Could you check a few things on this model? Use its own coordinates, in mm. A direction names the side the tool comes from. Give positions to 0.01 mm unless a question says otherwise; leave off trailing zeros. Write each loop counter-clockwise with the first axis right and the second up, starting at its lowest first coordinate (ties: lowest second). Pieces come first, ordered by that corner, then holes. Notation, with made-up numbers: (-16, -18) -> (38, -18) arc R18 ccw to (38, -4) -> close; hole circle Ø8 at (31, 80.25). An arc over 180 degrees is marked (long way). Write item = value, one per line. Start each with the question number.
```python
from build123d import *

# Parameters (mm, degrees)
F1_DEPTH = 19.05
F3_DEPTH = 4
F4_R     = 1.55
F5_DEPTH = 2.5


with BuildPart() as f1:
    # F0 (on Top) → F1 (new body)
    with BuildSketch(Plane.XY):
        with BuildLine():
            Line((12.7, 0), (11.7422761358, 0))
            ThreePointArc((11.7422761358, 0), (14.5035288799, 0.4316708576), (15.774, 2.921))
            ThreePointArc((15.774, 2.921), (14.5035288799, 5.4103291424), (11.7422761358, 5.842))
            Line((11.7422761358, 5.842), (12.7, 5.842))
            Line((12.7, 5.842), (12.7, 4.471))
            ThreePointArc((12.7, 4.471), (13.7960155108, 4.0170155108), (14.25, 2.921))
            ThreePointArc((14.25, 2.921), (13.7960155108, 1.8249844892), (12.7, 1.371))
            Line((12.7, 1.371), (12.7, 0))
        make_face()
        with BuildLine():
            Line((0, 1.524), (0, 0))
            Line((0, 0), (11.7422761358, 0))
            ThreePointArc((11.7422761358, 0), (9.626, 2.921), (11.7422761358, 5.842))
            Line((11.7422761358, 5.842), (0, 5.842))
            Line((0, 5.842), (0, 4.318))
            Line((0, 4.318), (8.89, 4.318))
            Line((8.89, 4.318), (8.89, 1.524))
            Line((8.89, 1.524), (0, 1.524))
        make_face()
        with BuildLine():
            ThreePointArc((11.7422761358, 5.842), (9.626, 2.921), (11.7422761358, 0))
            Line((11.7422761358, 0), (12.7, 0))
            Line((12.7, 0), (12.7, 1.371))
            ThreePointArc((12.7, 1.371), (11.15, 2.921), (12.7, 4.471))
            Line((12.7, 4.471), (12.7, 5.842))
            Line((12.7, 5.842), (11.7422761358, 5.842))
        make_face()
    extrude(amount=F1_DEPTH)

    # F2 (on face) → F3 (join)
    with BuildSketch(Plane.XY.offset(19.05)):
        with BuildLine():
            ThreePointArc((10.2538072439, 0), (14.3118476354, -0.5312524821), (16.51, 2.921))
            ThreePointArc((16.51, 2.921), (14.3118476354, 6.3732524821), (10.2538072439, 5.842))
            Line((10.2538072439, 5.842), (11.7422761358, 5.842))
            ThreePointArc((11.7422761358, 5.842), (15.774, 2.921), (11.7422761358, 0))
            Line((11.7422761358, 0), (10.2538072439, 0))
        make_face()
    extrude(amount=-F3_DEPTH)

    # F4 (on face) → F5 (cut)
    with BuildSketch(Plane.XY.offset(19.05)):
        Polygon((15.45, 4.5087132403), (12.7, 6.0964264805), (9.95, 4.5087132403), (9.95, 1.3332867597), (12.7, -0.2544264805), (15.45, 1.3332867597), align=None)
        with Locations((12.7, 2.921)):
            Circle(F4_R, mode=Mode.SUBTRACT)
    extrude(amount=-F5_DEPTH, mode=Mode.SUBTRACT)


solid = f1.part
```
(1) Imagine slicing it at D-D (y = 5). Please give me the cut outline in (x, z).
(2) Imagine slicing it at A-A (z = 13.25). Please give me the cut outline in (x, y).
(3) We'd pull the mould along Y, two halves only. Please class faces 4 (the flat face through (0, 1, 9)), 5 (the flat face through (4, 4.318, 9)), 6 (the flat face through (6, 5.842, 9)): released by +Y, released by -Y, zero draft, split by the parting line, or undercut.
(4) On a 3-axis mill with a long thin cutter (end or side, diameter ignored), from which of +Z, -Z, +X, -X, +Y, -Y can I reach the whole of each face in a straight line? I mean faces 1 (the flat face through (8.89, 3, 9)), 2 (the flat face through (10, 3, 0)), 3 (the flat face through (15.45, 3, 18)). Say none if no direction works.
(5) If I drill on line 1 along Y through (x, z) = (3.5, 6.75); line 2 along Y through (x, z) = (12.75, 3.5); line 3 along Z through (x, y) = (15.25, 4.25), over which ranges is the centre line in solid material (lowest first)? Write a range as from..to.
(6) Imagine slicing it at B-B (x = 3.25). Please give me the cut outline in (y, z).
(7) I'm going to push flat-ended pins straight in: pin 1 (4.5 mm diameter, centred on x = 5, z = 9.5, fed in from -Y); pin 2 (1 mm diameter, centred on x = 12, y = 1, fed in from +Z); pin 3 (8 mm diameter, centred on x = 8, z = 7, fed in from +Y). Where does each tip first touch, or does it pass through?
(8) Imagine slicing it at C-C (z = 17.75). Please give me the cut outline in (x, y), then the cut area to 3 significant figures.
Answers below:
q1.outline = (0, 0) -> (14.96, 0) -> (14.96, 15.05) -> (15.89, 15.05) -> (15.89, 19.05) -> (14.6, 19.05) -> (14.6, 16.55) -> (10.8, 16.55) -> (10.8, 19.05) -> (0, 19.05) -> close
q2.outline = (0, 0) -> (11.74, 0) arc R3.07 ccw (long way) to (11.74, 5.84) -> (0, 5.84) -> (0, 4.32) -> (8.89, 4.32) -> (8.89, 1.52) -> (0, 1.52) -> close; hole circle Ø3.1 at (12.7, 2.92)
q3.face_4 = zero draft
q3.face_5 = undercut
q3.face_6 = released by +Y
q4.face_1 = +Z, -Z, -X
q4.face_2 = -Z, +X, -X, +Y, -Y
q4.face_3 = +Z
q5.line_1 = 0..1.52, 4.32..5.84
q5.line_2 = -0.15..1.37, 4.47..5.99
q5.line_3 = 0..16.55
q6.outline = (0, 0) -> (1.52, 0) -> (1.52, 19.05) -> (0, 19.05) -> close; (4.32, 0) -> (5.84, 0) -> (5.84, 19.05) -> (4.32, 19.05) -> close
q7.pin_1 = 0
q7.pin_2 = 16.55
q7.pin_3 = 5.91
q8.outline = (0, 0) -> (10.25, 0) arc R3.81 ccw (long way) to (10.25, 5.84) -> (0, 5.84) -> (0, 4.32) -> (8.89, 4.32) -> (8.89, 1.52) -> (0, 1.52) -> close; hole (9.95, 1.33) -> (12.7, -0.25) -> (15.45, 1.33) -> (15.45, 4.51) -> (12.7, 6.1) -> (9.95, 4.51) -> close
q8.area = 48.9 mm^2
